Can you work these out from the model? Positions are in its coordinate system, mm. Give positions to 0.01 mm unless a question says otherwise; leave off trailing zeros. Order: outer loops, then holes, each group sorted by start corner. A loop starts at its lowest first (then second) coordinate and runs counter-clockwise, first axis right, second up. Notation, with made-up numbers: (7.5, -5.5) - (58.5, -5.5) arc R26 ccw to (58.5, 30.5) - close; hole circle Ø4 at (-0.5, 31.25). An arc over 180 degrees is marked (long way). One line per question, with ' | ' between items.
```python
from build123d import *

# Parameters (mm, degrees)
SKETCH1_R             = 18
BOSS_EXTRUDE1_DEPTH   = 2
F_2_0MM_DOWEL_HOLE1_D = 2
SKETCH5_R             = 1.2
CUT_EXTRUDE4_DEPTH    = 42.060930335


with BuildPart() as part:
    # Sketch1 → Boss-Extrude1 (new body)
    with BuildSketch(Plane.XY):
        with BuildLine():
            ThreePointArc((-29, 0), (0, -29), (29, 0))
            ThreePointArc((29, 0), (0, 29), (-29, 0))
        make_face()
        Circle(SKETCH1_R, mode=Mode.SUBTRACT)
    extrude(amount=BOSS_EXTRUDE1_DEPTH)

    # Ø2.0mm Dowel Hole1 (through all)
    with Locations(Plane(origin=(-19, 19, 2), x_dir=(1, 0, 0), z_dir=(0, 0, 1))):
        with Locations((0, 0), (2, -2), (36, -2), (38, 0), (36, -36), (38, -38), (0, -38), (2, -36)):
            Hole(F_2_0MM_DOWEL_HOLE1_D / 2)

    # Sketch5 → Cut-Extrude4 (cut, through all)
    with BuildSketch(Plane.XY):
        with Locations((-12.5, 21.650635095)):
            Circle(SKETCH5_R)
        with Locations((-25, 0)):
            Circle(SKETCH5_R)
        with Locations((25, 0)):
            Circle(SKETCH5_R)
        with Locations((-12.5, -21.650635095)):
            Circle(SKETCH5_R)
        with Locations((12.5, 21.650635095)):
            Circle(SKETCH5_R)
        with Locations((12.5, -21.650635095)):
            Circle(SKETCH5_R)
    extrude(amount=CUT_EXTRUDE4_DEPTH, mode=Mode.SUBTRACT)


solid = part.part
```
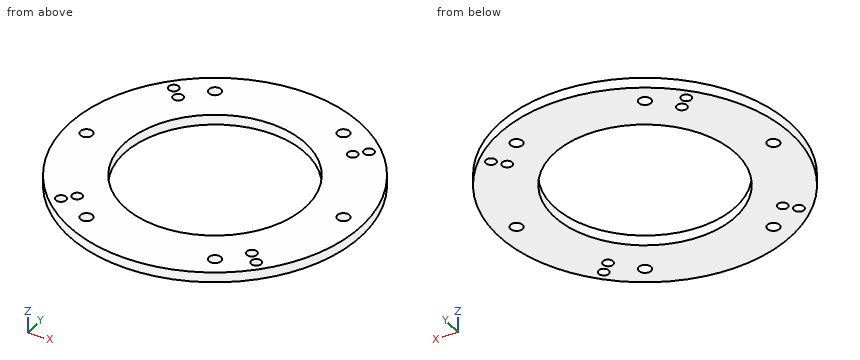
(1) Imagine slicing it at D-D (z = 0.9). Count the separate pieces of the cut face and the enclosed holes in it, and give its area (3 significant figures).
Answer below:
separate pieces: 1 | enclosed holes: 15 | area: 1,570 mm^2
(2) If I drill on line 1 (Y direction, x = -19, z = 1.2); line 2 (Y direction, x = 12.5, z = 1); line 3 (X direction, y = -8, z = 0.9), over which ranges is the centre line in solid material (lowest first)?
Answer below:
line 1: -21.91 to -20, -18 to 18, 20 to 21.91 | line 2: -26.17 to -22.85, -20.45 to -12.95, 12.95 to 20.45, 22.85 to 26.17 | line 3: -27.87 to -16.12, 16.12 to 27.87
(3) Imagine slicing it at C-C (y = -12.5). List the corners of the cut face in (x, z) for me, and give its area (3 significant figures).
Answer below:
outline: (-26.17, 0) - (-12.95, 0) - (-12.95, 2) - (-26.17, 2) - close; (12.95, 0) - (26.17, 0) - (26.17, 2) - (12.95, 2) - close | area: 52.9 mm^2
(4) Imagine slicing it at B-B (x = -1.5). List the corners of the cut face in (y, z) for me.
Answer below:
outline: (-28.96, 0) - (-17.94, 0) - (-17.94, 2) - (-28.96, 2) - close; (17.94, 0) - (28.96, 0) - (28.96, 2) - (17.94, 2) - close
(5) Will these pins go through, and if not, where does the flat tip stop? pin 1 (1.4 mm diameter, centred on x = -12.5, y = -21.65, fed in from -Z); pin 2 (1 mm diameter, centred on y = 18.5, z = 1, fed in from +X).
Answer below:
pin 1: through | pin 2: x = 22.74
(6) Imagine slicing it at A-A (y = 0). List the corners of the cut face in (x, z) for me, and give its area (3 significant figures).
Answer below:
outline: (-29, 0) - (-26.2, 0) - (-26.2, 2) - (-29, 2) - close; (-23.8, 0) - (-18, 0) - (-18, 2) - (-23.8, 2) - close; (18, 0) - (23.8, 0) - (23.8, 2) - (18, 2) - close; (26.2, 0) - (29, 0) - (29, 2) - (26.2, 2) - close | area: 34.4 mm^2
